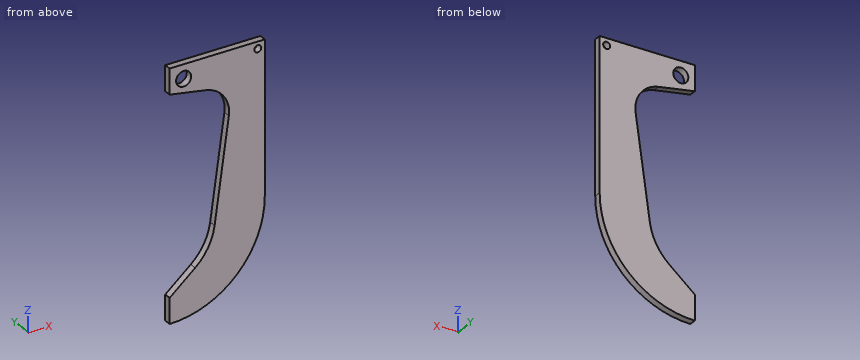
```python
from build123d import *

# Parameters (mm, degrees)
SKETCH1_R           = 3.429
SKETCH1_R_2         = 1.5875
BOSS_EXTRUDE1_DEPTH = 3.175
CUT_EXTRUDE1_DEPTH  = 120.85362166


with BuildPart() as part:
    # Sketch1 → Boss-Extrude1 (new body)
    with BuildSketch(Plane(origin=(0, 0, 0), x_dir=(1, 0, 0), z_dir=(0, 1, 0))):
        with BuildLine():
            Line((0, 0), (43.18, 0))
            Line((43.18, 0), (43.18, 68.58))
            ThreePointArc((43.18, 68.58), (30.532870812, 99.112870812), (0, 111.76))
            Line((0, 111.76), (0, 0))
        make_face()
        with Locations(Location((6.35, 6.35, 0), (0, 0, 270))):
            Circle(SKETCH1_R, mode=Mode.SUBTRACT)
        with Locations(Location((40.005, 3.175, 0), (0, 0, 270))):
            Circle(SKETCH1_R_2, mode=Mode.SUBTRACT)
    extrude(amount=BOSS_EXTRUDE1_DEPTH)

    # Sketch2 → Cut-Extrude1 (cut, through all)
    with BuildSketch(Plane(origin=(0, 3.175, 0), x_dir=(1, 0, 0), z_dir=(0, 1, 0))):
        with BuildLine():
            Line((16.499594236, 14.339323634), (0, 11.43))
            Line((0, 11.43), (0, 100.33))
            Line((0, 100.33), (11.578626407, 90.614378852))
            ThreePointArc((11.578626407, 90.614378852), (17.468445655, 83.468697719), (20.405366763, 74.686600928))
            Line((20.405366763, 74.686600928), (26.8710352, 28.611257563))
            ThreePointArc((26.8710352, 28.611257563), (24.567999732, 19.380438031), (16.499594236, 14.339323634))
        make_face()
    extrude(amount=-CUT_EXTRUDE1_DEPTH, mode=Mode.SUBTRACT)


solid = part.part
```
Build history of the part. All positions in model axes, mm. Round coordinates to 2 decimals unless told otherwise and drop trailing zeros. Order: outer loops, then holes, each group sorted by start corner. A loop starts at its lowest first (then second) coordinate and runs counter-clockwise, first axis right, second up. Notation, with made-up numbers: (73.5, 82) -> (113.5, 82) arc R25 cw to (113.5, 117) -> close; hole circle Ø2 at (14.5, -36.5). An arc over 180 degrees is marked (long way). Answer in a Markdown table with one row per item.
1) Band-saw the part on A-A on z = -6.35. Give the cut face in (x, y) (3 decimals), and give its area (3 significant figures).
Values:
| item | result |
|---|---|
| outline | (0, 0) -> (2.921, 0) -> (2.921, 3.175) -> (0, 3.175) -> close; (9.779, 0) -> (43.18, 0) -> (43.18, 3.175) -> (9.779, 3.175) -> close |
| area | 115 mm2 |
2) Pin check, flat tips, straight feed: P1, Ø1.5, axis at y = 1, z = -57.5, coming from the -X side; P2, Ø1.5, axis at y = 2, z = -84.5, coming from the +X side. Stop position of each tip, or through.
Values:
| item | result |
|---|---|
| P1 | x = 22.71 |
| P2 | x = 40.43 |
3) Wall check: L1, parallel to Z at x = 9, y = 2.1; L2, parallel to X at y = 1.5, z = -6.35; L3, parallel to Z at x = 5, y = 0.3. Give the ranges that are in metal, low to high.
Values:
| item | result |
|---|---|
| L1 | -110.81 to -92.78, -13.02 to -8.53, -4.17 to 0 |
| L2 | 0 to 2.92, 9.78 to 43.18 |
| L3 | -111.47 to -96.13, -12.31 to -9.5, -3.2 to 0 |
4) Band-saw the part on B-B on x = 14. Give the cut face in (y, z) (3 decimals), and give its area (3 significant figures).
Values:
| item | result |
|---|---|
| outline | (0, -109.427) -> (3.175, -109.427) -> (3.175, -88.294) -> (0, -88.294) -> close; (0, -13.899) -> (3.175, -13.899) -> (3.175, 0) -> (0, 0) -> close |
| area | 111 mm2 |
5) Band-saw the part on C-C on y = 1.6. Give the number of separate pieces and of enclosed holes in the cut face, and give its area (3 significant figures).
Values:
| item | result |
|---|---|
| separate pieces | 1 |
| enclosed holes | 2 |
| area | 2,580 mm2 |
6) Band-saw the part on D-D on x = 8. Give the cut face in (y, z) (3 decimals), and give its area (3 significant figures).
Values:
| item | result |
|---|---|
| outline | (0, -111.012) -> (3.175, -111.012) -> (3.175, -93.617) -> (0, -93.617) -> close; (0, -12.841) -> (3.175, -12.841) -> (3.175, -9.356) -> (0, -9.356) -> close; (0, -3.344) -> (3.175, -3.344) -> (3.175, 0) -> (0, 0) -> close |
| area | 76.9 mm2 |
